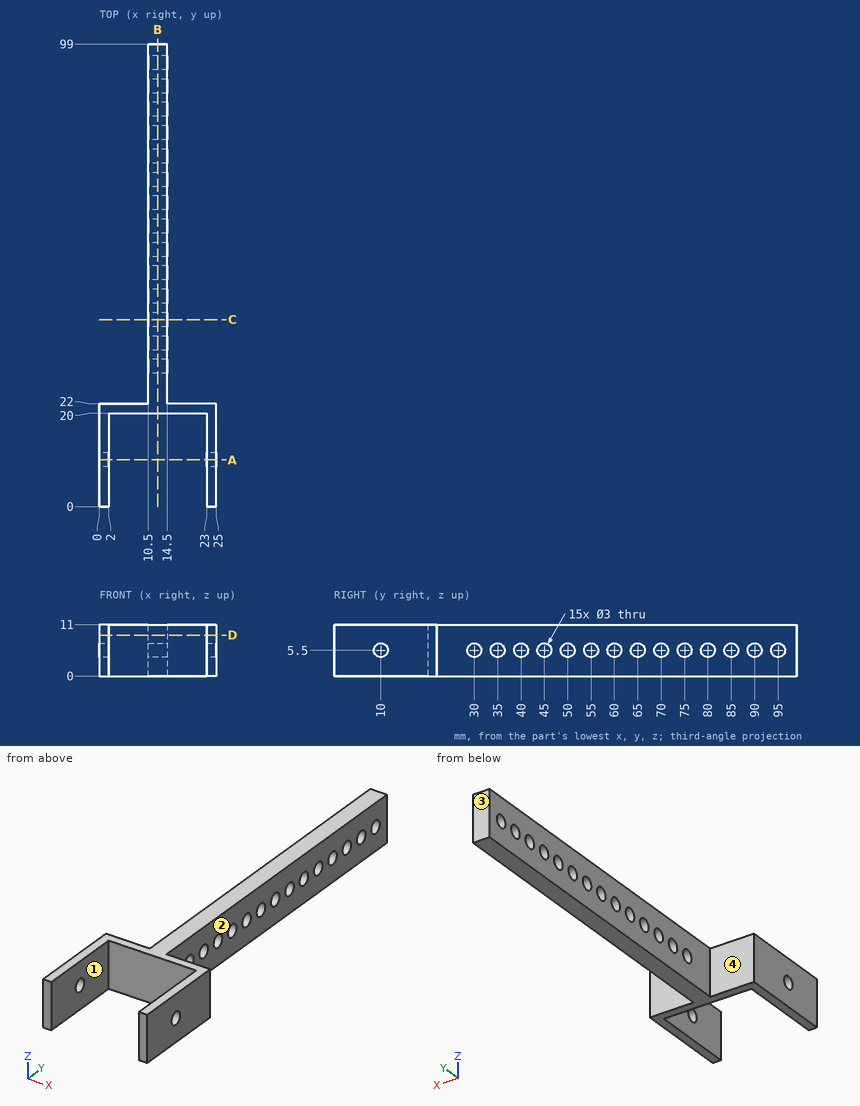
Here's the drawing with two shaded views (mm, measured from the low corner). I have some questions. A direction names the side the tool comes from. Coordinates: 2 decimals unless noted, no trailing zeros. Write each loop counter-clockwise with the first axis right and the second up, starting at its lowest first coordinate (ties: lowest second). Pieces come first, ordered by that corner, then holes. Notation, with made-up numbers: (-18, 61) -> (40, 61) arc R8 ccw to (40, 74) -> close; hole circle Ø1 at (71.5, -19). An arc over 180 degrees is marked (long way). One line per question, with ' | ' between items. Start each with the question number.
1. If we section it at C-C (y = 40): Please give me the cut outline in (x, z), and give its area (3 significant figures).
2. Will these pins go through, and if not, where does the flat tip stop? P1, Ø5.5, axis at x = 10, z = 6.5, coming from the -Y side; P2, Ø5.5, axis at y = 54, z = 4.5, coming from the +X side; P3, Ø4, axis at y = 34.5, z = 5.5, coming from the -X side; P4, Ø2.5, axis at y = 65, z = 5.5, coming from the +X side.
3. For the marked faces 1, 2, 3 and 4, which set-ups out of +Z, -Z, +X, -X, +Y, -Y let a thin tool reach every point of the face, with its end or its side?
4. If we section it at D-D (z = 8.75): Please give me the cut outline in (x, y).
5. If we section it at B-B (x = 12.5): Count the separate pieces of the cut face and the enclosed holes in it, and give its area (3 significant figures).
6. If we section it at A-A (y = 10): Please give me the cut outline in (x, z), and give its area (3 significant figures).
7. Please list where these lines run through material, in increasing order: line 1 along Z through (x, y) = (11.6, 95); line 2 along Y through (x, z) = (1.5, 3.5); line 3 along X through (y, z) = (56, 10).
Return value:
1) outline: (10.5, 0) -> (14.5, 0) -> (14.5, 4) -> (10.5, 4) -> close; (10.5, 7) -> (14.5, 7) -> (14.5, 11) -> (10.5, 11) -> close | area: 32.0 mm²
2) P1: stops at y = 20 | P2: stops at x = 14.5 | P3: stops at x = 10.5 | P4: passes through
3) face 1: +Z, -Z, -Y | face 2: +Z, -Z, +X, +Y | face 3: +Z, -Z, +X, -X, +Y | face 4: +Z, -Z, -X, +Y
4) outline: (0, 0) -> (2, 0) -> (2, 20) -> (23, 20) -> (23, 0) -> (25, 0) -> (25, 22) -> (14.5, 22) -> (14.5, 99) -> (10.5, 99) -> (10.5, 22) -> (0, 22) -> close
5) separate pieces: 1 | enclosed holes: 14 | area: 770 mm²
6) outline: (0, 0) -> (2, 0) -> (2, 4) -> (0, 4) -> close; (0, 7) -> (2, 7) -> (2, 11) -> (0, 11) -> close; (23, 0) -> (25, 0) -> (25, 4) -> (23, 4) -> close; (23, 7) -> (25, 7) -> (25, 11) -> (23, 11) -> close | area: 32.0 mm²
7) line 1: z = 0 to 4, 7 to 11 | line 2: y = 0 to 22 | line 3: x = 10.5 to 14.5
